Geometry: see drawing. Coordinates: mm, zero at the bounding-box minimum. A direction names the side the tool comes from. Round coordinates to 2 decimals unless told otherwise and drop trailing zeros. Order: outer loops, then holes, each group sorted by start corner. A loop starts at its lowest first (then second) coordinate and runs counter-clockwise, first axis right, second up. Notation, with made-up numbers: (53, -13) -> (83, -13) arc R26 ccw to (83, 1) -> close; hole circle Ø9 at (44.5, 67.5). An arc over 180 degrees is marked (long way). One line per item, written item: value. Start each with the question number.
1) Ray query, L1, parallel to X at y = 18, z = 5.5 (1 decimal); L2, parallel to X at y = 66, z = 3.25 (1 decimal); L3, parallel to Y at x = 17.75, z = 2.75 (1 decimal). Return the intervals inside material, ascending.
2) Section B-B (x = 10). Return the cut outline in (y, z), and give its area (3 significant figures).
3) Reachability of the marked faces 4, 5, 6, 7 and 8 from +Z, -Z, +X, -X, +Y, -Y: full face, straight path, thin tool, end or side. Return the list, or none.
4) Section C-C (y = 65.5). Return the cut outline in (x, z).
5) Mould query, pull axis X, two halves, no side actions, for the marked faces 1, 2 and 3. Classes: pulls with the +X half, pulls with the -X half, needs draft (parallel to the pull), parting line crosses it, or undercut.
6) Pin query (flat end, axial travel): P1, Ø3.5, axis at y = 47, z = 4.5, coming from the +X side (1 decimal); P2, Ø3.5, axis at y = 45.5, z = 4.5, coming from the -X side (1 decimal); P3, Ø3.5, axis at y = 1, z = 5, coming from the -X side (1 decimal). Return the tip coordinate at first contact, or that it passes through.
7) Section A-A (y = 11.5). Return the cut outline in (x, z) (1 decimal), and give its area (3 significant figures).
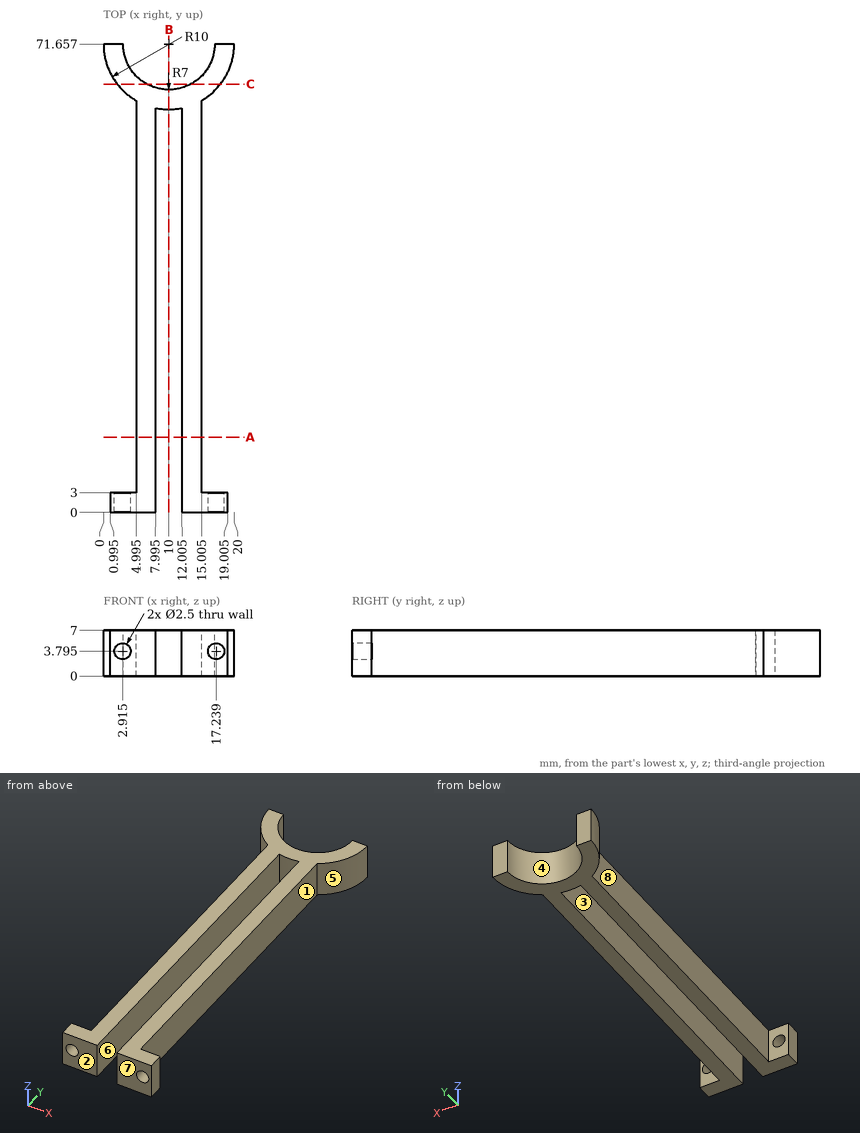
Findings:
1. L1: 5 to 8, 12 to 15
1. L2: 1.8 to 5.9, 14.1 to 18.2
1. L3: 65.3 to 71.7
2. outline: (61.66, 0) -> (64.66, 0) -> (64.66, 7) -> (61.66, 7) -> close
2. area: 21.0 mm2
3. face 4: +Z, -Z, +Y
3. face 5: +Z, -Z, +X
3. face 6: +Z, -Z, -Y
3. face 7: +Z, -Z, +X, -X, -Y
3. face 8: +Z, -Z, -X
4. outline: (2.12, 0) -> (6.67, 0) -> (6.67, 7) -> (2.12, 7) -> close; (13.33, 0) -> (17.88, 0) -> (17.88, 7) -> (13.33, 7) -> close
5. face 1: pulls with the +X half
5. face 2: needs draft
5. face 3: undercut
6. P1: x = 15
6. P2: x = 5
6. P3: x = 1
7. outline: (5, 0) -> (8, 0) -> (8, 7) -> (5, 7) -> close; (12, 0) -> (15, 0) -> (15, 7) -> (12, 7) -> close
7. area: 42.0 mm2
